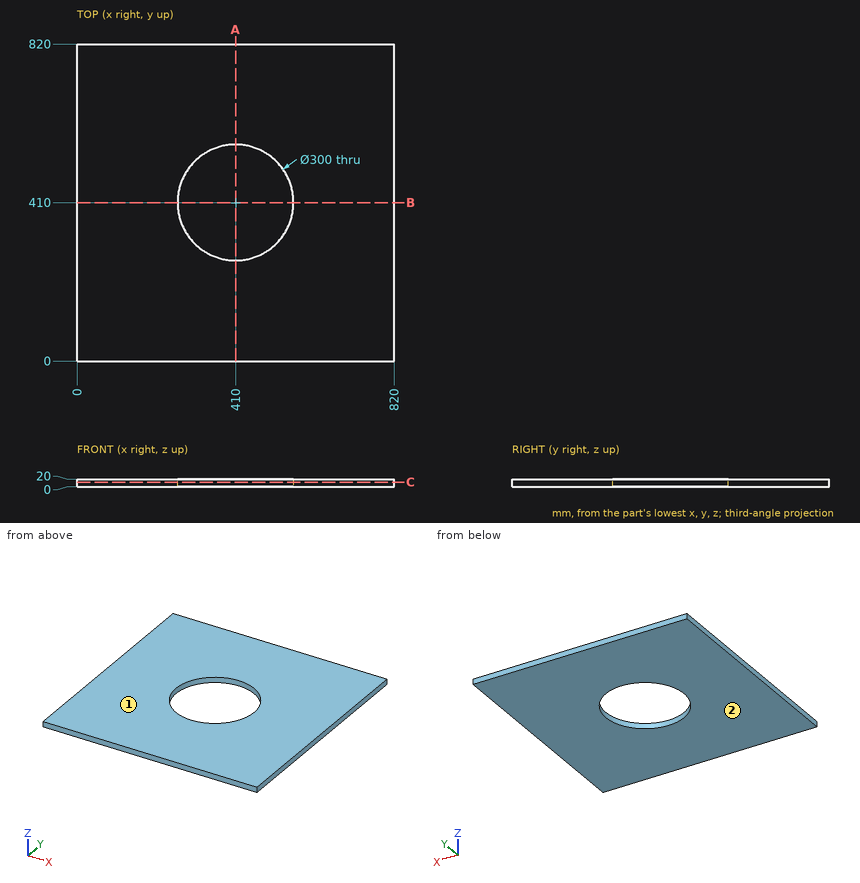
Study the drawing (mm; zero at the part's minimum x, y, z) and answer. Give positions to 0.01 mm unless a question says otherwise; leave off trailing zeros. Order: outer loops, then holes, each group sorted by start corner. A loop starts at its lowest first (then second) coordinate and runs counter-clockwise, first axis right, second up.
1. Section A-A, the plane x = 410 is taken. Determine the outline of the cut face in (y, z).
Result sheet:
outline: (0, 0) - (260, 0) - (260, 20) - (0, 20) - close; (560, 0) - (820, 0) - (820, 20) - (560, 20) - close
2. Section C-C, the plane z = 11.75 is taken. Determine the outline of the cut face in (x, y), and give its area (3 significant figures).
Result sheet:
outline: (0, 0) - (820, 0) - (820, 820) - (0, 820) - close; hole circle Ø300 at (410, 410)
area: 602,000 mm2
3. Straight lines are drawn through the part: L1, parallel to Y at x = 410, z = 6.5; L2, parallel to Y at x = 302, z = 10.25; L3, parallel to X at y = 533, z = 10.25. For each, find the intervals that lie inside material, in ascending order.
Result sheet:
L1: y = 0 to 260, 560 to 820
L2: y = 0 to 305.9, 514.1 to 820
L3: x = 0 to 324.15, 495.85 to 820
4. The mould has two halves that part along Z. Classify the marked faces 1 and 2: released by +Z, released by -Z, zero draft, split by the parting line, or undercut.
Result sheet:
face 1: released by +Z
face 2: released by -Z
